Print and shaded views of the part. All mm, measured from the part's lowest x, y and z. A direction names the side the tool comes from. Coordinates: 2 decimals unless noted, no trailing zeros. Write each loop counter-clockwise with the first axis right and the second up, starting at its lowest first coordinate (ties: lowest second). Pieces come first, ordered by that corner, then holes. Notation, with made-up numbers: (85, 7.25) -> (118, 7.25) arc R14 cw to (118, 32.25) -> close; hole circle Ø2 at (-16.75, -30). An arc over 180 degrees is marked (long way). Write item = value, one per line.
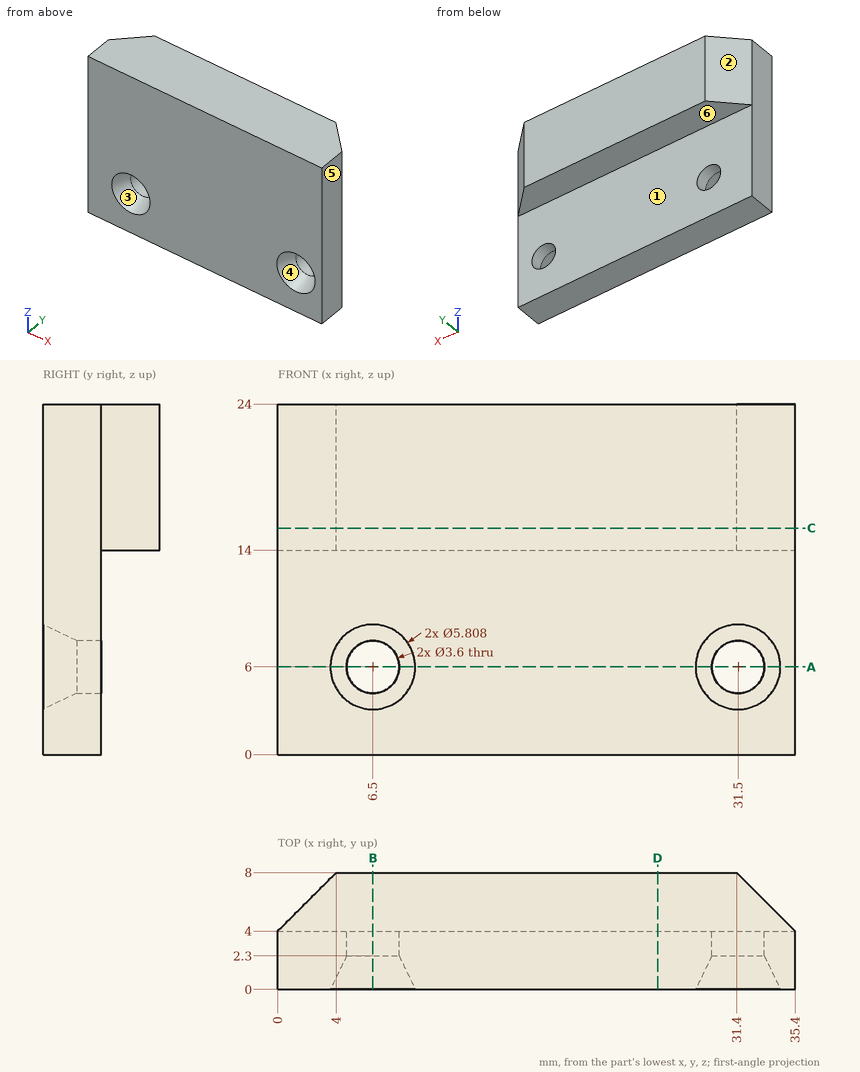
Q1. Saw through at B-B on x = 6.5. Give the cut face in (y, z), and give its area (3 significant figures).
Model answer:
outline = (0, 0) -> (4, 0) -> (4, 4.2) -> (2.3, 4.2) -> (0, 3.1) -> close; (0, 8.9) -> (2.3, 7.8) -> (4, 7.8) -> (4, 14) -> (8, 14) -> (8, 24) -> (0, 24) -> close
area = 119 mm²
Q2. Pin check, flat tips, straight feed: pin 1 (6 mm diameter, centred on x = 6.5, z = 6, fed in from +Y); pin 2 (8 mm diameter, centred on x = 25, z = 10.5, fed in from +Y); pin 3 (3 mm diameter, centred on x = 31.5, z = 6, fed in from +Y); pin 4 (4.5 mm diameter, centred on x = 26, y = 6.5, fed in from -Z). Stop position of each tip, or through.
Model answer:
pin_1 = 4
pin_2 = 8
pin_3 = through
pin_4 = 14
Q3. Mould opens along X. For the marked faces 1, 2, 3 and 4 say: released by +X, released by -X, zero draft, split by the parting line, or undercut.
Model answer:
face_1 = zero draft
face_2 = released by -X
face_3 = undercut
face_4 = undercut
Q4. Probe line 1 (X direction, y = 2.9, z = 6); line 2 (Y direction, x = 23, z = 6); line 3 (Z direction, x = 4.5, y = 7.25). List the from-to ranges inside material, lowest first. Write a range as from..to.
Model answer:
line_1 = 0..4.7, 8.3..29.7, 33.3..35.4
line_2 = 0..4
line_3 = 14..24
Q5. Which spindle directions (+Z, -Z, +X, -X, +Y, -Y) get a long thin tool onto all of the face, cutting with end or side? Do the marked faces 5 and 6. Say none if no direction does.
Model answer:
face_5 = +Z, -Z, +X, +Y, -Y
face_6 = -Z, +X, -X, +Y
Q6. Saw through at C-C on z = 15.5. Give the cut face in (x, y).
Model answer:
outline = (0, 0) -> (35.4, 0) -> (35.4, 4) -> (31.4, 8) -> (4, 8) -> (0, 4) -> close
Q7. Saw through at A-A on z = 6. Give the cut face in (x, y), and give its area (3 significant figures).
Model answer:
outline = (0, 0) -> (3.6, 0) -> (4.7, 2.3) -> (4.7, 4) -> (0, 4) -> close; (8.3, 2.3) -> (9.4, 0) -> (28.6, 0) -> (29.7, 2.3) -> (29.7, 4) -> (8.3, 4) -> close; (33.3, 2.3) -> (34.4, 0) -> (35.4, 0) -> (35.4, 4) -> (33.3, 4) -> close
area = 108 mm²
Q8. Saw through at D-D on x = 26. Give the cut face in (y, z), and give its area (3 significant figures).
Model answer:
outline = (0, 0) -> (4, 0) -> (4, 14) -> (8, 14) -> (8, 24) -> (0, 24) -> close
area = 136 mm²
